Source: CAD feature listing. Evaluate the final solid. Frame: model axes, mm. Round coordinates to 2 decimals unless told otherwise and drop trailing zeros. Loops run counter-clockwise (first coordinate to the right, second up) from the corner with the lowest first, then second, coordinate; pieces in that order, holes last. Notation, with made-up numbers: (-14.75, 43) - (1.25, 43) arc R9 cw to (1.25, 52) - close; hole circle Ø1 at (30.5, -17). An arc over 180 degrees is marked (long way). One line per question, with ' | ' between items.
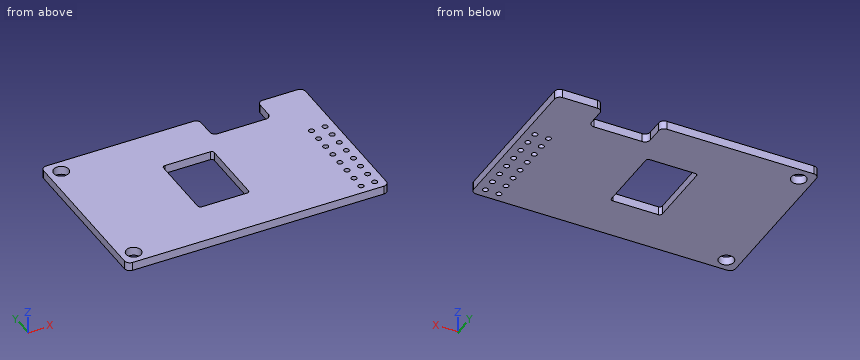
from build123d import *

# Parameters (mm, degrees)
SKETCH001_W         = 49
SKETCH001_H         = 31
SKETCH001_W_2       = 9.5
SKETCH001_H_2       = 13.25
PAD_DEPTH           = 1.6
SKETCH002_R         = 0.5
HOLE_DEPTH          = 25
LINEARPATTERN_COUNT = 8
LINEARPATTERN_PITCH = 2.54
SKETCH003_W         = 11
SKETCH003_H         = 5
POCKET_DEPTH        = 1.601
SKETCH004_R         = 1.4
HOLE001_DEPTH       = 25
FILLET_R            = 1
FILLET001_R         = 0.5
FILLET002_R         = 1


with BuildPart() as part:
    # Sketch001 → Pad (new body)
    with BuildSketch(Plane.XY):
        with Locations((-24.5, 15.5)):
            Rectangle(SKETCH001_W, SKETCH001_H)
        with Locations((-26.25, 15.375)):
            Rectangle(SKETCH001_W_2, SKETCH001_H_2, mode=Mode.SUBTRACT)
    extrude(amount=PAD_DEPTH)

    # Sketch002 (on Face10 of Pad) → Hole (cut)
    with BuildSketch(Plane.XY.offset(1.6)):
        with Locations((-1.78, 1.78)):
            Circle(SKETCH002_R)
        with Locations((-4.32, 1.78)):
            Circle(SKETCH002_R)
    hole = extrude(amount=-HOLE_DEPTH, mode=Mode.SUBTRACT)

    # LinearPattern: Hole ×8
    with Locations(*[(0, i * LINEARPATTERN_PITCH, 0) for i in range(1, LINEARPATTERN_COUNT)]):
        add(hole, mode=Mode.SUBTRACT)

    # Sketch003 (on Face5 of LinearPattern) → Pocket (cut, through all)
    with BuildSketch(Plane.XY.offset(1.6)):
        with Locations((-14, 28.5)):
            Rectangle(SKETCH003_W, SKETCH003_H)
    extrude(amount=-POCKET_DEPTH, mode=Mode.SUBTRACT)

    # Sketch004 (on Face5 of Pocket) → Hole001 (cut)
    with BuildSketch(Plane.XY.offset(1.6)):
        with Locations((-46.5, 28.5)):
            Circle(SKETCH004_R)
        with Locations((-46.5, 2.5)):
            Circle(SKETCH004_R)
    extrude(amount=-HOLE001_DEPTH, mode=Mode.SUBTRACT)

    # Fillet
    fillet_edges = [part.edges().sort_by_distance(p)[0] for p in [
        (-8.5, 26, 0.8),
        (-19.5, 26, 0.8),
        (-19.5, 31, 0.8),
        (-8.5, 31, 0.8),
        (0, 31, 0.8),
        (0, 0, 0.8),
    ]]
    fillet(fillet_edges, radius=FILLET_R)

    # Fillet001
    fillet001_edges = [part.edges().sort_by_distance(p)[0] for p in [
        (-21.5, 22, 0.8),
        (-21.5, 8.75, 0.8),
        (-31, 8.75, 0.8),
        (-31, 22, 0.8),
    ]]
    fillet(fillet001_edges, radius=FILLET001_R)

    # Fillet002
    fillet002_edges = [part.edges().sort_by_distance(p)[0] for p in [
        (-49, 31, 0.8),
        (-49, 0, 0.8),
    ]]
    fillet(fillet002_edges, radius=FILLET002_R)


solid = part.part
1. Section query B-B, the plane y = 19.56. Return loops of the section in (x, z), plus the area to 3 significant figures.
Worked out:
outline: (-49, 0) - (-31, 0) - (-31, 1.6) - (-49, 1.6) - close; (-21.5, 0) - (-4.82, 0) - (-4.82, 1.6) - (-21.5, 1.6) - close; (-3.82, 0) - (-2.28, 0) - (-2.28, 1.6) - (-3.82, 1.6) - close; (-1.28, 0) - (0, 0) - (0, 1.6) - (-1.28, 1.6) - close | area: 60.0 mm2
2. Section query A-A, the plane x = -30. Return loops of the section in (y, z).
Worked out:
outline: (0, 0) - (8.75, 0) - (8.75, 1.6) - (0, 1.6) - close; (22, 0) - (31, 0) - (31, 1.6) - (22, 1.6) - close
3. Section query C-C, the plane y = 28.5. Return loops of the section in (x, z).
Worked out:
outline: (-49, 0) - (-47.9, 0) - (-47.9, 1.6) - (-49, 1.6) - close; (-45.1, 0) - (-19.5, 0) - (-19.5, 1.6) - (-45.1, 1.6) - close; (-8.5, 0) - (0, 0) - (0, 1.6) - (-8.5, 1.6) - close
4. Contact query for flat-ended pins moving along their axis: P1, Ø0.5, axis at x = -12, z = 0.5, coming from the +Y side; P2, Ø2, axis at x = -46.5, y = 2.5, coming from the +Z side. Output: stop coordinate, or through.
Worked out:
P1: stops at y = 26 | P2: passes through
5. Section query D-D, the plane y = 10.5. Return loops of the section in (x, z), plus the area to 3 significant figures.
Worked out:
outline: (-49, 0) - (-31, 0) - (-31, 1.6) - (-49, 1.6) - close; (-21.5, 0) - (0, 0) - (0, 1.6) - (-21.5, 1.6) - close | area: 63.2 mm2
6. Material intervals for probe 1 along X at (y, z) = (12, 1.5); probe 2 along X at (y, z) = (11.5, 0.7); probe 3 along X at (y, z) = (29.5, 1.3), sorted ascending.
Worked out:
probe 1: x = -49 to -31, -21.5 to -4.82, -3.82 to -2.28, -1.28 to 0 | probe 2: x = -49 to -31, -21.5 to -4.56, -4.08 to -2.02, -1.54 to 0 | probe 3: x = -49 to -47.48, -45.52 to -19.5, -8.5 to 0
